For this review, take the finished solid that the model builds, in its own axes (mm). Face numbers are marked on the shaded views. A direction names the side the tool comes from. Coordinates: 2 decimals unless noted, no trailing zeros. Loops run counter-clockwise (first coordinate to the right, second up) from the corner with the lowest first, then second, coordinate; pieces in that order, holes last.
1. To check wall thickness, follow probe 1 along X at (y, z) = (3.25, 1); probe 2 along Z at (x, y) = (8, 6.5); probe 3 along X at (y, z) = (-6.5, 2.65). State the ranges of each line that lie inside material, in increasing order.
2. Take a section at A-A, the plane y = 0. State the section outline as (x, z) points.
3. Machinability: for the marked faces 4, 5 and 6, which of the approach directions +Z, -Z, +X, -X, +Y, -Y give a long, thin tool a straight path to every point of the face, cutting with its end or side? Answer none if there is none.
4. Mouldability with a two-part tool opening along X and no side actions: class the marked faces 1, 2 and 3 as pulls with the +X half, pulls with the -X half, needs draft (parallel to the pull), parting line crosses it, or undercut.
5. Take a section at C-C, the plane y = -6.5. Count the separate pieces of the cut face and the enclosed holes in it, then the cut area to 3 significant figures.
6. Take a section at B-B, the plane z = 12.25. State the section outline as (x, y) points.
7. Take a section at D-D, the plane z = 15. State the section outline as (x, y) points.
8. Clearance check with flat-ended pins moving along their axes: P1, Ø5, axis at x = -3, z = 12, coming from the +Y side; P2, Ø3.5, axis at x = -5.63, y = 3.25, coming from the +Z side; P3, Ø4, axis at x = -1, y = 13, coming from the +Z side. State where each tip first meets the part, or that it passes through.
```python
from build123d import *

# Parameters (mm, degrees)
F0_R     = 11.25
F1_DEPTH = 4
F2_R     = 4.5
F3_DEPTH = 6
F6_R     = 2
F7_DEPTH = 4


with BuildPart() as f1:
    # F0 (on Top) → F1 (new body)
    with BuildSketch(Plane.XY):
        Circle(F0_R)
    extrude(amount=F1_DEPTH)

    # F2 (on face) → F3 (join)
    with BuildSketch(Plane.XY.offset(4)):
        Circle(F2_R)
    extrude(amount=F3_DEPTH)

    # F4 (on Front) → F5 (revolve)
    with BuildSketch(Plane.XZ):
        with BuildLine():
            Line((3, 14), (0, 14))
            Line((0, 14), (0, 10))
            Line((0, 10), (4.5, 10))
            Line((4.5, 10), (26.5, 21))
            ThreePointArc((26.5, 21), (25.5, 22), (24.5, 21))
            Line((24.5, 21), (3, 14))
        make_face()
    revolve(axis=Axis((0, 0, 19.201497), (0, 0, 1)))

    # F6 (on face) → F7 (cut, through all)
    with BuildSketch(Plane(origin=(0, 0, 0), x_dir=(1, 0, 0), z_dir=(0, 0, -1))):
        with Locations((-5.629165, -3.25)):
            Circle(F6_R)
        with Locations((5.629165, -3.25)):
            Circle(F6_R)
        with Locations((0, 6.5)):
            Circle(F6_R)
    extrude(amount=-F7_DEPTH, mode=Mode.SUBTRACT)


solid = f1.part
```
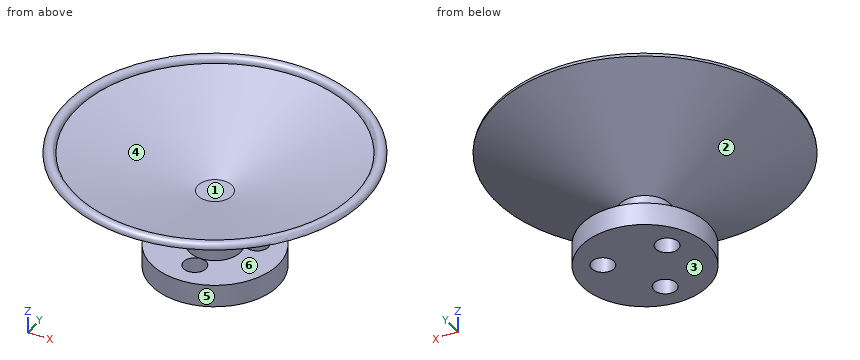
Results list:
1. probe 1: x = -10.77 to -7.63, -3.63 to 3.63, 7.63 to 10.77
1. probe 2: z = 0 to 4, 12.9 to 16.38
1. probe 3: x = -9.18 to -2, 2 to 9.18
2. outline: (-26.5, 21) - (-4.5, 10) - (-4.5, 4) - (-11.25, 4) - (-11.25, 0) - (11.25, 0) - (11.25, 4) - (4.5, 4) - (4.5, 10) - (26.5, 21) arc R1 ccw to (24.5, 21) - (3, 14) - (-3, 14) - (-24.5, 21) arc R1 ccw to start
3. face 4: +Z
3. face 5: -Z
3. face 6: none
4. face 1: undercut
4. face 2: parting line crosses it
4. face 3: needs draft
5. separate pieces: 3
5. enclosed holes: 0
5. area: 196 mm2
6. outline: circle Ø18 at (0, 0)
7. outline: circle Ø29 at (0, 0); hole circle Ø12.14 at (0, 0)
8. P1: stops at y = 13.19
8. P2: stops at z = 15.71
8. P3: stops at z = 17.92
